The model under review builds one solid part; all positions refer to its coordinate system, in mm. A direction names the side the tool comes from. Coordinates: 2 decimals unless noted, no trailing zeros. Write each loop counter-clockwise with the first axis right and the second up, starting at its lowest first coordinate (ties: lowest second). Pieces come first, ordered by that corner, then holes. Notation, with made-up numbers: (36.5, 11.5) - (48.5, 11.5) arc R9 cw to (48.5, 15.5) - close; hole circle Ø10 at (-18, 52). An arc over 180 degrees is marked (long way). Put each result on its own line as item: value.
from build123d import *

# Parameters (mm, degrees)
F0_W     = 2
F0_H     = 19.5
F1_DEPTH = 21.9
F2_W     = 19.5
F2_H     = 2.5
F3_DEPTH = 40.4
F0_R     = 1.75
F4_DEPTH = 3
F5_R     = 3


with BuildPart() as f1:
    # F0 (on Top) → F1 (new body)
    with BuildSketch(Plane.XY):
        Polygon((-24.159199, 0), (-24.159199, 19.5), (-26.159199, 19.5), (-26.159199, 9.75), (-26.159199, 0), align=None)
        with Locations((17.240801, 9.75)):
            Rectangle(F0_W, F0_H)
    extrude(amount=F1_DEPTH)

    # F2 (on face) → F3 (join, through all)
    with BuildSketch(Plane(origin=(16.240801, 0, 0), x_dir=(0, -1, 0), z_dir=(-1, 0, 0))):
        with Locations((-9.75, 20.65)):
            Rectangle(F2_W, F2_H)
    extrude(amount=F3_DEPTH)

    # F0 (on Top) → F4 (join)
    with BuildSketch(Plane.XY):
        Polygon((-26.159199, 9.75), (-26.159199, 19.5), (-28.959199, 19.5), (-31.959199, 19.5), (-31.959199, 0), (-28.959199, 0), (-26.159199, 0), align=None)
        with Locations((-28.959199, 4.75)):
            Circle(F0_R, mode=Mode.SUBTRACT)
        with Locations((-28.959199, 9.75)):
            Circle(F0_R, mode=Mode.SUBTRACT)
        with Locations((-28.959199, 14.75)):
            Circle(F0_R, mode=Mode.SUBTRACT)
        Polygon((21.040801, 19.5), (18.240801, 19.5), (18.240801, 0), (21.040801, 0), (24.040801, 0), (24.040801, 19.5), align=None)
        with Locations((21.040801, 4.75)):
            Circle(F0_R, mode=Mode.SUBTRACT)
        with Locations((21.040801, 9.75)):
            Circle(F0_R, mode=Mode.SUBTRACT)
        with Locations((21.040801, 14.75)):
            Circle(F0_R, mode=Mode.SUBTRACT)
    extrude(amount=F4_DEPTH)

    # F5
    f5_edges = [f1.edges().sort_by_distance(p)[0] for p in [
        (18.240801, 9.75, 21.9),
        (-26.159199, 9.75, 21.9),
        (24.040801, 0, 1.5),
        (24.040801, 19.5, 1.5),
        (-31.959199, 19.5, 1.5),
        (-31.959199, 0, 1.5),
    ]]
    fillet(f5_edges, radius=F5_R)


solid = f1.part
1. For pin 1 Ø5.5 at (x, y) = (21.04, 9.75) entering from +Z; pin 2 Ø8 at (x, z) = (-16.5, 9.5) entering from -Y; pin 3 Ø6.5 at (x, y) = (20.5, 10) entering from +Z; pin 4 Ø6 at (y, z) = (13, 8) entering from +X, all flat-tipped, find the tip position at first contact; note any pin that passes through.
Determined:
pin 1: stops at z = 3
pin 2: passes through
pin 3: stops at z = 21.13
pin 4: stops at x = 18.24
2. Consider section A-A on z = 7.75. State the section outline as (x, y) points, plus the area to 3 significant figures.
Determined:
outline: (-26.16, 0) - (-24.16, 0) - (-24.16, 19.5) - (-26.16, 19.5) - close; (16.24, 0) - (18.24, 0) - (18.24, 19.5) - (16.24, 19.5) - close
area: 78.0 mm^2
3. Machinability: for faces 1 (the flat face through (-27, 10, 3)), 2 (the flat face through (19, 10, 3)), 3 (the flat face through (-24.159, 10, 10)), which of the approach directions +Z, -Z, +X, -X, +Y, -Y give a long, thin tool a straight path to every point of the face, cutting with its end or side? Answer none if there is none.
Determined:
face 1: +Z, -X, +Y, -Y
face 2: +Z, +X, +Y, -Y
face 3: -Z, +Y, -Y
4. The part is to be moulded in two halves that separate along X. For faces 4 (the cylindrical face through (-31.1, 0.9, 1.5)), 5 (the cylindrical face through (17.339, 9.886, 21.045)), 6 (the flat face through (-26, 10, 0)), 7 (the cylindrical face through (-29.187, 11.485, 1.479)), say which applies: +X half, -X half, draft (parallel to the pull), parting line (faces both ways), or undercut.
Determined:
face 4: -X half
face 5: +X half
face 6: draft
face 7: undercut
5. Consider section C-C on x = 20.5. State the section outline as (y, z) points.
Determined:
outline: (0, 0) - (3.09, 0) - (3.09, 3) - (0, 3) - close; (6.41, 0) - (8.09, 0) - (8.09, 3) - (6.41, 3) - close; (11.41, 0) - (13.09, 0) - (13.09, 3) - (11.41, 3) - close; (16.41, 0) - (19.5, 0) - (19.5, 3) - (16.41, 3) - close
6. Consider section D-D on x = 14.5. State the section outline as (y, z) points.
Determined:
outline: (0, 19.4) - (19.5, 19.4) - (19.5, 21.9) - (0, 21.9) - close
7. Consider section B-B on y = 9.75. State the section outline as (x, z) points.
Determined:
outline: (-31.96, 0) - (-30.71, 0) - (-30.71, 3) - (-31.96, 3) - close; (-27.21, 0) - (-24.16, 0) - (-24.16, 19.4) - (16.24, 19.4) - (16.24, 0) - (19.29, 0) - (19.29, 3) - (18.24, 3) - (18.24, 18.9) arc R3 ccw to (15.24, 21.9) - (-23.16, 21.9) arc R3 ccw to (-26.16, 18.9) - (-26.16, 3) - (-27.21, 3) - close; (22.79, 0) - (24.04, 0) - (24.04, 3) - (22.79, 3) - close
8. To check wall thickness, follow probe 1 along X at (y, z) = (3.5, 6.5); probe 2 along Z at (x, y) = (-20.5, 10.75); probe 3 along Z at (x, y) = (-24.5, 16). State the ranges of each line that lie inside material, in increasing order.
Determined:
probe 1: x = -26.16 to -24.16, 16.24 to 18.24
probe 2: z = 19.4 to 21.9
probe 3: z = 0 to 21.58
